```python
from build123d import *

# Parameters (mm, degrees)
F0_R     = 76.2
F1_DEPTH = 12.7


with BuildPart() as f1:
    # F0 (on Top) → F1 (new body)
    with BuildSketch(Plane.XY):
        Circle(F0_R)
        with BuildLine():
            ThreePointArc((47.0895163427, 42.6007916665), (58.6663503145, 24.3003979552), (63.420625, 3.1740076574))
            ThreePointArc((63.420625, 3.1740076574), (65.7168231069, 2.2729540938), (66.675, 0))
            ThreePointArc((66.675, 0), (65.7168231069, -2.2729540938), (63.420625, -3.1740076574))
            ThreePointArc((63.420625, -3.1740076574), (58.6663503145, -24.3003979552), (47.0895163427, -42.6007916665))
            ThreePointArc((47.0895163427, -42.6007916665), (47.8191799753, -43.6496863153), (48.0762806053, -44.9012806053))
            ThreePointArc((48.0762806053, -44.9012806053), (46.0795362268, -47.8495578465), (42.6007916665, -47.0895163427))
            ThreePointArc((42.6007916665, -47.0895163427), (24.3003979552, -58.6663503145), (3.1740076574, -63.420625))
            ThreePointArc((3.1740076574, -63.420625), (3.1747519047, -63.4603093986), (3.175, -63.5))
            ThreePointArc((3.175, -63.5), (-0.0396906014, -66.6747519047), (-3.1740076574, -63.420625))
            ThreePointArc((-3.1740076574, -63.420625), (-24.3003979552, -58.6663503145), (-42.6007916665, -47.0895163427))
            ThreePointArc((-42.6007916665, -47.0895163427), (-47.1463446356, -47.1463446356), (-47.0895163427, -42.6007916665))
            ThreePointArc((-47.0895163427, -42.6007916665), (-58.6663503145, -24.3003979552), (-63.420625, -3.1740076574))
            ThreePointArc((-63.420625, -3.1740076574), (-66.675, 0), (-63.420625, 3.1740076574))
            ThreePointArc((-63.420625, 3.1740076574), (-58.6663503145, 24.3003979552), (-47.0895163427, 42.6007916665))
            ThreePointArc((-47.0895163427, 42.6007916665), (-47.1463446356, 47.1463446356), (-42.6007916665, 47.0895163427))
            ThreePointArc((-42.6007916665, 47.0895163427), (-24.3003979552, 58.6663503145), (-3.1740076574, 63.420625))
            ThreePointArc((-3.1740076574, 63.420625), (-0.0396906014, 66.6747519047), (3.175, 63.5))
            ThreePointArc((3.175, 63.5), (3.1747519047, 63.4603093986), (3.1740076574, 63.420625))
            ThreePointArc((3.1740076574, 63.420625), (24.3003979552, 58.6663503145), (42.6007916665, 47.0895163427))
            ThreePointArc((42.6007916665, 47.0895163427), (46.0795362268, 47.8495578465), (48.0762806053, 44.9012806053))
            ThreePointArc((48.0762806053, 44.9012806053), (47.8191799753, 43.6496863153), (47.0895163427, 42.6007916665))
        make_face(mode=Mode.SUBTRACT)
        with BuildLine():
            Line((0, 0), (42.6562165751, 42.6562165751))
            ThreePointArc((42.6562165751, 42.6562165751), (41.7265287007, 44.8615900039), (42.6007916665, 47.0895163427))
            ThreePointArc((42.6007916665, 47.0895163427), (24.3003979552, 58.6663503145), (3.1740076574, 63.420625))
            ThreePointArc((3.1740076574, 63.420625), (0, 60.325), (-3.1740076574, 63.420625))
            ThreePointArc((-3.1740076574, 63.420625), (-24.3003979552, 58.6663503145), (-42.6007916665, 47.0895163427))
            ThreePointArc((-42.6007916665, 47.0895163427), (-41.9530033642, 46.0795362268), (-41.7262806053, 44.9012806053))
            ThreePointArc((-41.7262806053, 44.9012806053), (-41.9679630896, 43.6862607076), (-42.6562165751, 42.6562165751))
            Line((-42.6562165751, 42.6562165751), (0, 0))
        make_face()
        with BuildLine():
            Line((-42.6562165751, -42.6562165751), (0, 0))
            Line((0, 0), (-42.6562165751, 42.6562165751))
            ThreePointArc((-42.6562165751, 42.6562165751), (-44.8615900039, 41.7265287007), (-47.0895163427, 42.6007916665))
            ThreePointArc((-47.0895163427, 42.6007916665), (-58.6663503145, 24.3003979552), (-63.420625, 3.1740076574))
            ThreePointArc((-63.420625, 3.1740076574), (-61.2270459062, 2.2168231069), (-60.325, 0))
            ThreePointArc((-60.325, 0), (-61.2270459062, -2.2168231069), (-63.420625, -3.1740076574))
            ThreePointArc((-63.420625, -3.1740076574), (-58.6663503145, -24.3003979552), (-47.0895163427, -42.6007916665))
            ThreePointArc((-47.0895163427, -42.6007916665), (-44.8615900039, -41.7265287007), (-42.6562165751, -42.6562165751))
        make_face()
        with BuildLine():
            ThreePointArc((42.6007916665, -47.0895163427), (41.7265287007, -44.8615900039), (42.6562165751, -42.6562165751))
            Line((42.6562165751, -42.6562165751), (0, 0))
            Line((0, 0), (-42.6562165751, -42.6562165751))
            ThreePointArc((-42.6562165751, -42.6562165751), (-41.9679630896, -43.6862607076), (-41.7262806053, -44.9012806053))
            ThreePointArc((-41.7262806053, -44.9012806053), (-41.9530033642, -46.0795362268), (-42.6007916665, -47.0895163427))
            ThreePointArc((-42.6007916665, -47.0895163427), (-24.3003979552, -58.6663503145), (-3.1740076574, -63.420625))
            ThreePointArc((-3.1740076574, -63.420625), (0, -60.325), (3.1740076574, -63.420625))
            ThreePointArc((3.1740076574, -63.420625), (24.3003979552, -58.6663503145), (42.6007916665, -47.0895163427))
        make_face()
        with BuildLine():
            ThreePointArc((63.420625, -3.1740076574), (60.325, 0), (63.420625, 3.1740076574))
            ThreePointArc((63.420625, 3.1740076574), (58.6663503145, 24.3003979552), (47.0895163427, 42.6007916665))
            ThreePointArc((47.0895163427, 42.6007916665), (44.8615900039, 41.7265287007), (42.6562165751, 42.6562165751))
            Line((42.6562165751, 42.6562165751), (0, 0))
            Line((0, 0), (42.6562165751, -42.6562165751))
            ThreePointArc((42.6562165751, -42.6562165751), (44.8615900039, -41.7265287007), (47.0895163427, -42.6007916665))
            ThreePointArc((47.0895163427, -42.6007916665), (58.6663503145, -24.3003979552), (63.420625, -3.1740076574))
        make_face()
    extrude(amount=F1_DEPTH)


solid = f1.part
```
CAD build for the part. Positions are in the model's coordinates, mm. Coordinates: 2 decimals unless noted, no trailing zeros. Loops run counter-clockwise (first coordinate to the right, second up) from the corner with the lowest first, then second, coordinate; pieces in that order, holes last. Notation, with made-up numbers: (81, 80) - (131, 80) arc R24 ccw to (131, 96) - close; hole circle Ø4 at (-10.5, 41.25). An arc over 180 degrees is marked (long way). Use CSV: the item, a comma, the result in double quotes. Start each with the question number.
Q1. Cut at B-B, the plane x = -39.5. List the corners of the cut face in (y, z).
Q2. Cut at A-A, the plane z = 9.5. State how many separate pieces and enclosed holes the cut face has, then the cut area to 3 significant figures.
Q3. Probe probe 1 along X at (y, z) = (-65, 11.5); probe 2 along X at (y, z) = (-45, 11.25); probe 3 along X at (y, z) = (-5.5, 10.75). List the from-to ranges inside material, lowest first. Write a range as from..to.
Q4. Cut at C-C, the plane y = -19.5. List the corners of the cut face in (x, z), then the cut area to 3 significant figures.
Q5. Drop flat-ended pins along their axis: P1, Ø5, axis at x = -26.5, z = 10, coming from the -Y side; P2, Ø6, axis at x = 16, z = 11, coming from the -Y side; P3, Ø3, axis at x = -59, z = 2.5, coming from the +Y side. Give the stop position or say it passes through.
Here are the results:
1,outline,"(-65.16, 0) - (65.16, 0) - (65.16, 12.7) - (-65.16, 12.7) - close"
2,separate pieces,"1"
2,enclosed holes,"8"
2,area,"18,000 mm2"
3,probe 1,"-39.77..-2.8, 2.8..39.77"
3,probe 2,"-61.49..-48.07, -41.73..41.73, 48.07..61.49"
3,probe 3,"-76..76"
4,outline,"(-73.66, 0) - (73.66, 0) - (73.66, 12.7) - (-73.66, 12.7) - close"
4,area,"1,870 mm2"
5,P1,"y = -72.32"
5,P2,"y = -75.08"
5,P3,"y = 50"
